Can you work these out from the model? Positions are in its coordinate system, mm. A direction names the side the tool comes from. Give positions to 0.01 mm unless a question says otherwise; leave off trailing zeros. Order: outer loops, then holes, each group sorted by start corner. A loop starts at its lowest first (then second) coordinate and runs counter-clockwise, first axis right, second up. Notation, with made-up numbers: M 54.25,-36 L 94.25,-36 A14 cw 94.25,-21 Z; hole C 50,-19 d9. An arc over 180 degrees is marked long. Use one line per item in the form item = value. Start each with the question number.
1. Will these pins go through, and if not, where does the flat tip stop? P1, Ø1.9, axis at x = 67, z = 3.5, coming from the +Y side; P2, Ø1.9, axis at y = -41.5, z = 3.5, coming from the -X side; P3, Ø3, axis at x = 22, z = 3.5, coming from the -Y side.
2. I want a section at A-A, the plane z = 4.75. List the corners of the cut face in (x, y) for me, and give its area (3 significant figures).
3. I want a section at B-B, the plane x = 22.5. List the corners of the cut face in (y, z) for me.
4. I want a section at C-C, the plane x = 60.5. List the corners of the cut face in (y, z) for me.
5. I need wall thicknesses on L1, parallel to Y at x = 31, z = 6.25; L2, parallel to Y at x = 22, z = 5; L3, parallel to X at y = -39, z = 1.75. Which ranges of each line are inside material? Lowest first, please.
6. For faces 1 (the face through (24.756, -9, 3)), 2 (the face through (18.406, -24, 3)), 3 (the face through (63, -37.27, 3)), 4 (the face through (31.106, -40, 3)), 5 (the face through (62.856, -9, 3)), which set-ups out of +Z, -Z, +X, -X, +Y, -Y let a thin tool reach every point of the face, with its end or its side?
```python
from build123d import *

# Parameters (mm, degrees)
F0_W     = 38.1
F0_H     = 38.1
F1_DEPTH = 6.35
F2_W     = 25.4
F2_H     = 6.35
F4_DEPTH = 6.35
F3_W     = 25.4
F3_H     = 6.35
F5_DEPTH = 6.35
F6_DEPTH = 6.35
F7_DEPTH = 6.35


with BuildPart() as f1:
    # F0 (on Top) → F1 (new body)
    with BuildSketch(Plane.XY):
        with Locations((43.8062495112, -24.5695395887)):
            Rectangle(F0_W, F0_H)
    extrude(amount=F1_DEPTH)

    # F2 (on face) → F4 (join)
    with BuildSketch(Plane.YZ.offset(62.8562495112)):
        with Locations((-24.5695395887, 3.175)):
            Rectangle(F2_W, F2_H)
    extrude(amount=F4_DEPTH)

    # F3 (on face) → F5 (join)
    with BuildSketch(Plane(origin=(24.7562495112, 0, 0), x_dir=(0, -1, 0), z_dir=(-1, 0, 0))):
        with Locations((24.5695395887, 3.175)):
            Rectangle(F3_W, F3_H)
    extrude(amount=F5_DEPTH)

    # F6 (cut): a face of the model
    f6_faces = [f1.faces().sort_by_distance(p)[0] for p in [
        (62.8562495112, -40.4445395887, 3.175),
    ]]
    extrude(f6_faces, amount=-F6_DEPTH, mode=Mode.SUBTRACT)

    # F7 (cut): a face of the model
    f7_faces = [f1.faces().sort_by_distance(p)[0] for p in [
        (24.7562495112, -40.4445395887, 3.175),
    ]]
    extrude(f7_faces, amount=-F7_DEPTH, mode=Mode.SUBTRACT)


solid = f1.part
```
Check result:
q1.P1 = -11.87
q1.P2 = 31.11
q1.P3 = -37.27
q2.outline = M 18.41,-37.27 L 31.11,-37.27 L 31.11,-43.62 L 56.51,-43.62 L 56.51,-37.27 L 69.21,-37.27 L 69.21,-11.87 L 62.86,-11.87 L 62.86,-5.52 L 24.76,-5.52 L 24.76,-11.87 L 18.41,-11.87 Z
q2.area = 1,690 mm2
q3.outline = M -37.27,0 L -11.87,0 L -11.87,6.35 L -37.27,6.35 Z
q4.outline = M -37.27,0 L -5.52,0 L -5.52,6.35 L -37.27,6.35 Z
q5.L1 = -37.27 to -5.52
q5.L2 = -37.27 to -11.87
q5.L3 = 31.11 to 56.51
q6.face_1 = +Z, -Z, -X, +Y
q6.face_2 = +Z, -Z, -X, +Y, -Y
q6.face_3 = +Z, -Z, +X, -Y
q6.face_4 = +Z, -Z, -X, -Y
q6.face_5 = +Z, -Z, +X, +Y
